```python
from build123d import *

# Parameters (mm, degrees)
F0_R     = 3.175
F1_DEPTH = 25.4
F2_R     = 2.38125
F3_DEPTH = 3.175
F4_W     = 12.7
F4_H     = 8.382
F5_DEPTH = 12.701
F6_SIZE2 = 0.79375
F6_SIZE  = 3.175


with BuildPart() as f1:
    # F0 (on Front) → F1 (new body)
    with BuildSketch(Plane.XZ):
        with BuildLine():
            Line((228.6, 0), (6.35, 0))
            ThreePointArc((6.35, 0), (3.175, -11.849261314), (11.849261314, -3.175))
            Line((11.849261314, -3.175), (228.6, -3.175))
            Line((228.6, -3.175), (228.6, 0))
        make_face()
        with Locations((6.35, -6.35)):
            Circle(F0_R, mode=Mode.SUBTRACT)
    extrude(amount=F1_DEPTH)

    # F2 (on face) → F3 (cut, through all)
    with BuildSketch(Plane.XY):
        with Locations((203.2, -12.7)):
            Circle(F2_R)
        with Locations((114.3, -12.7)):
            Circle(F2_R)
        with Locations((25.4, -12.7)):
            Circle(F2_R)
    extrude(amount=-F3_DEPTH, mode=Mode.SUBTRACT)

    # F4 (on face) → F5 (cut, through all)
    with BuildSketch(Plane.XY):
        with Locations((6.35, -12.573)):
            Rectangle(F4_W, F4_H)
    extrude(amount=-F5_DEPTH, mode=Mode.SUBTRACT)

    # F6
    f6_edges = [f1.edges().sort_by_distance(p)[0] for p in [
        (120.224631, -25.4, -3.175),
        (120.224631, 0, -3.175),
        (228.6, -12.7, -3.175),
    ]]
    f6_side = f1.faces().sort_by_distance((120.424157, -12.700166, -3.175))[0]
    chamfer(f6_edges, length=F6_SIZE, length2=F6_SIZE2, reference=f6_side)


solid = f1.part
```
Could you check a few things on this model? Use its own coordinates, in mm. A direction names the side the tool comes from. Coordinates: 2 decimals unless noted, no trailing zeros. Write each loop counter-clockwise with the first axis right and the second up, starting at its lowest first coordinate (ties: lowest second). Pieces come first, ordered by that corner, then holes. Notation, with made-up numbers: (74, 65.25) -> (107, 65.25) arc R27 cw to (107, 101.25) -> close; hole circle Ø4 at (4, -4). An arc over 180 degrees is marked (long way). Return JSON: item names as keys, results as strings.
(1) Imagine slicing it at D-D, the plane x = 71. Please give me the cut outline in (y, z) (3 decimals), then the cut area to 3 significant figures.
Numbers:
{"outline": "(-25.4, -2.381) -> (-22.225, -3.175) -> (-3.175, -3.175) -> (0, -2.381) -> (0, 0) -> (-25.4, 0) -> close", "area": "78.1 mm2"}
(2) Which directions (+Z, -Z, +X, -X, +Y, -Y) give clear straight access to the entire face, cutting with the end or side of a thin tool? Please do faces 1 (the flat face through (97, 0, -2)), 2 (the flat face through (8, -8.382, -3)).
Numbers:
{"face 1": "+Z, -Z, +X, -X, +Y", "face 2": "+Z, -Z, -X"}
(3) Imagine slicing it at B-B, the plane z = -6.35. Please give me the cut outline in (x, y) (3 decimals).
Numbers:
{"outline": "(0, -25.4) -> (3.175, -25.4) -> (3.175, -16.764) -> (0, -16.764) -> close; (0, -8.382) -> (3.175, -8.382) -> (3.175, 0) -> (0, 0) -> close; (9.525, -25.4) -> (12.7, -25.4) -> (12.7, -16.764) -> (9.525, -16.764) -> close; (9.525, -8.382) -> (12.7, -8.382) -> (12.7, 0) -> (9.525, 0) -> close"}
(4) I'm going to push flat-ended pins straight in: pin 1 (4 mm diameter, centred on x = 6.35, z = -6.35, fed in from +Y); pin 2 (3 mm diameter, centred on y = -18, z = -11, fed in from -X); pin 3 (2.5 mm diameter, centred on y = -14, z = -1.5, fed in from -X); pin 4 (2 mm diameter, centred on x = 60.5, y = -22.5, fed in from -Z) (3 decimals). Where does each tip first touch, or does it pass through?
Numbers:
{"pin 1": "passes through", "pin 2": "stops at x = 0.84", "pin 3": "stops at x = 12.7", "pin 4": "stops at z = -3.175"}
(5) We'd pull the mould along Z, two halves only. Please class faces 3 (the flat face through (119, -13, 0)), 4 (the cylindrical face through (205.47, -11.98, -1.57)), 5 (the cylindrical face through (3.83, -4.13, -8.28)): +Z half, -Z half, draft (parallel to the pull), parting line (faces both ways), or undercut.
Numbers:
{"face 3": "+Z half", "face 4": "draft", "face 5": "undercut"}
(6) Imagine slicing it at A-A, the plane x = 203.2. Please give me the cut outline in (y, z) (3 decimals).
Numbers:
{"outline": "(-25.4, -2.381) -> (-22.225, -3.175) -> (-15.081, -3.175) -> (-15.081, 0) -> (-25.4, 0) -> close; (-10.319, -3.175) -> (-3.175, -3.175) -> (0, -2.381) -> (0, 0) -> (-10.319, 0) -> close"}
(7) Imagine slicing it at C-C, the plane y = -5.5. Please give me the cut outline in (x, z) (3 decimals), then the cut area to 3 significant figures.
Numbers:
{"outline": "(6.35, 0) arc R6.35 ccw (long way) to (11.849, -3.175) -> (225.425, -3.175) -> (228.6, -2.381) -> (228.6, 0) -> close; hole circle Ø6.35 at (6.35, -6.35)", "area": "787 mm2"}
(8) I need wall thicknesses on L1, parallel to X at y = -3.5, z = -6.35 (3 decimals); L2, parallel to Y at x = 203.2, z = -0.7; L3, parallel to Z at x = 6.35, y = -4 (3 decimals). Which ranges of each line are inside material? Lowest first, please.
Numbers:
{"L1": "x = 0 to 3.175, 9.525 to 12.7", "L2": "y = -25.4 to -15.08, -10.32 to 0", "L3": "z = -12.7 to -9.525, -3.175 to 0"}
